Check sheet for the modelled part. Datum: model origin and axes. Units: mm. Face numbers are marked on the shaded views. Coordinates: 2 decimals unless noted, no trailing zeros. Write each loop counter-clockwise with the first axis right and the second up, starting at its lowest first coordinate (ties: lowest second). Pieces come first, ordered by that corner, then holes. Notation, with made-up numbers: M 57.25,52.25 L 62.25,52.25 A17 cw 62.25,82.25 Z; hole C -4,29.25 d4. An arc over 180 degrees is marked long. Answer as CSV lines item,"result".
from build123d import *

# Parameters (mm, degrees)
SKETCH1_R           = 12.7
BOSS_EXTRUDE1_DEPTH = 82.55
SKETCH2_R           = 50.8
BOSS_EXTRUDE2_DEPTH = 0.508


with BuildPart() as part:
    # Sketch1 → Boss-Extrude1 (new body, symmetric)
    with BuildSketch(Plane(origin=(0, 0, 0), x_dir=(1, 0, 0), z_dir=(0, 1, 0))):
        Circle(SKETCH1_R)
    extrude(amount=BOSS_EXTRUDE1_DEPTH, both=True)

    # Sketch2 → Boss-Extrude2 (add)
    with BuildSketch(Plane(origin=(0, 82.55, 0), x_dir=(1, 0, 0), z_dir=(0, 1, 0))):
        Circle(SKETCH2_R)
    boss_extrude2 = extrude(amount=BOSS_EXTRUDE2_DEPTH)

    # Mirror1: Boss-Extrude2 across plane
    add(boss_extrude2.mirror(Plane.ZX))


solid = part.part
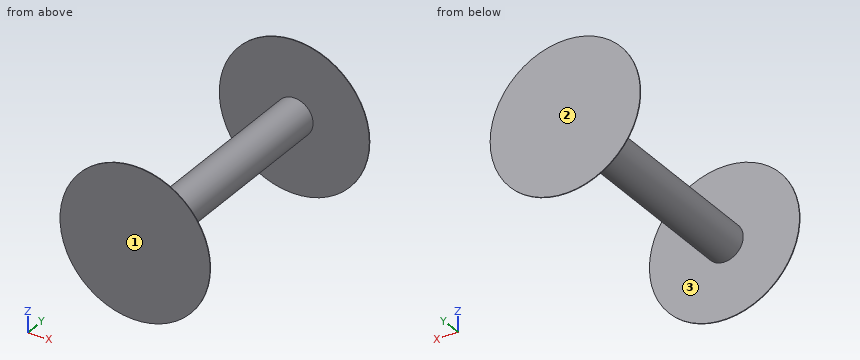
1) Thickness scan on line 1 along Y through (x, z) = (-22.5, 24); line 2 along Z through (x, y) = (-1, -9); line 3 along Z through (x, y) = (-11, 6.5). Record the ranges inside material, lowest first.
Answer key:
line 1,"y = -83.06 to -82.55, 82.55 to 83.06"
line 2,"z = -12.66 to 12.66"
line 3,"z = -6.35 to 6.35"
2) Section check C-C, the plane x = -36. Record the boundary of the cut face in (y, z), plus the area to 3 significant figures.
Answer key:
outline,"M -83.06,-35.84 L -82.55,-35.84 L -82.55,35.84 L -83.06,35.84 Z; M 82.55,-35.84 L 83.06,-35.84 L 83.06,35.84 L 82.55,35.84 Z"
area,"72.8 mm2"
3) Section check B-B, the plane z = -39.5. Record the boundary of the cut face in (x, y), plus the area to 3 significant figures.
Answer key:
outline,"M -31.94,-83.06 L 31.94,-83.06 L 31.94,-82.55 L -31.94,-82.55 Z; M -31.94,82.55 L 31.94,82.55 L 31.94,83.06 L -31.94,83.06 Z"
area,"64.9 mm2"
4) Section check D-D, the plane z = 0. Record the boundary of the cut face in (x, y).
Answer key:
outline,"M -50.8,-83.06 L 50.8,-83.06 L 50.8,-82.55 L 12.7,-82.55 L 12.7,82.55 L 50.8,82.55 L 50.8,83.06 L -50.8,83.06 L -50.8,82.55 L -12.7,82.55 L -12.7,-82.55 L -50.8,-82.55 Z"
5) Mould release check, pull along Y, two halves, no side actions. Record for the marked faces 1, 2 and 3: pulls with the +Y half, pulls with the -Y half, needs draft (parallel to the pull), parting line crosses it, or undercut.
Answer key:
face 1,"pulls with the -Y half"
face 2,"pulls with the +Y half"
face 3,"undercut"
6) Section check A-A, the plane x = 0. Record the boundary of the cut face in (y, z), plus the area to 3 significant figures.
Answer key:
outline,"M -83.06,-50.8 L -82.55,-50.8 L -82.55,-12.7 L 82.55,-12.7 L 82.55,-50.8 L 83.06,-50.8 L 83.06,50.8 L 82.55,50.8 L 82.55,12.7 L -82.55,12.7 L -82.55,50.8 L -83.06,50.8 Z"
area,"4,300 mm2"
